Here's how the part is built. I have some questions about the finished solid (model axes, mm). A direction names the side the tool comes from. Give positions to 0.01 mm unless a question says otherwise; leave off trailing zeros. Write each loop counter-clockwise with the first axis right and the second up, starting at its lowest first coordinate (ties: lowest second). Pieces come first, ordered by that corner, then holes. Notation, with made-up numbers: (36.25, 73) -> (53.25, 73) arc R34 cw to (53.25, 110) -> close; hole circle Ø1 at (8, -25.75). An arc over 180 degrees is marked (long way). Return JSON: item names as keys, results as strings.
from build123d import *

# Parameters (mm, degrees)
CROQUIS1_W              = 5.7
CROQUIS1_H              = 2.6
SALIENTE_EXTRUIR1_DEPTH = 6.2
CROQUIS2_W              = 5.4
CROQUIS2_H              = 0.8
SALIENTE_EXTRUIR2_DEPTH = 1.4
SALIENTE_EXTRUIR3_DEPTH = 1
MATRIZL1_COUNT          = 2
MATRIZL1_PITCH          = 4.2


with BuildPart() as part:
    # Croquis1 → Saliente-Extruir1 (new body)
    with BuildSketch(Plane(origin=(0, 0, 0), x_dir=(0, 0, -1), z_dir=(1, 0, 0))):
        with Locations((2.85, 1.3)):
            Rectangle(CROQUIS1_W, CROQUIS1_H)
    extrude(amount=SALIENTE_EXTRUIR1_DEPTH)

    # Croquis2 → Saliente-Extruir2 (add)
    with BuildSketch(Plane.XY):
        with Locations((3.1, 0.4)):
            Rectangle(CROQUIS2_W, CROQUIS2_H)
    extrude(amount=SALIENTE_EXTRUIR2_DEPTH)

    # Croquis3 → Saliente-Extruir3 (add)
    with BuildSketch(Plane.ZY.offset(-0.5)):
        Polygon((-5.7, 1.8), (-6.3, 1.8), (-7.167456635, 0.5), (-8.7, 0.5), (-8.7, 0), (-6.9, 0), (-6.032543365, 1.3), (-5.7, 1.3), align=None)
    saliente_extruir3 = extrude(amount=-SALIENTE_EXTRUIR3_DEPTH)

    # MatrizL1: Saliente-Extruir3 ×2
    with Locations(*[(i * MATRIZL1_PITCH, 0, 0) for i in range(1, MATRIZL1_COUNT)]):
        add(saliente_extruir3)


solid = part.part
1. Suppose I cut it at B-B, the plane y = 0.2. List the corners of the cut face in (x, z) for me, and give its area (3 significant figures).
Taken from the geometry:
{"outline": "(0, -5.7) -> (6.2, -5.7) -> (6.2, 0) -> (5.8, 0) -> (5.8, 1.4) -> (0.4, 1.4) -> (0.4, 0) -> (0, 0) -> close; (0.5, -8.7) -> (1.5, -8.7) -> (1.5, -6.77) -> (0.5, -6.77) -> close; (4.7, -8.7) -> (5.7, -8.7) -> (5.7, -6.77) -> (4.7, -6.77) -> close", "area": "46.8 mm²"}
2. For pin 1 Ø0.8 at (x, y) = (4.5, 2) entering from +Z; pin 2 Ø1.4 at (y, z) = (1, -8) entering from +X; pin 3 Ø0.6 at (y, z) = (0.5, 1) entering from +X; pin 4 Ø0.5 at (y, z) = (1.5, -7) entering from +X, each with a flat end and sliding along its axis, tell me the tip position at first contact or that it passes through.
Taken from the geometry:
{"pin 1": "stops at z = 0", "pin 2": "stops at x = 5.7", "pin 3": "stops at x = 5.8", "pin 4": "passes through"}
3. Suppose I cut it at A-A, the plane z = -7.75. List the corners of the cut face in (x, y) for me, and give its area (3 significant figures).
Taken from the geometry:
{"outline": "(0.5, 0) -> (1.5, 0) -> (1.5, 0.5) -> (0.5, 0.5) -> close; (4.7, 0) -> (5.7, 0) -> (5.7, 0.5) -> (4.7, 0.5) -> close", "area": "1.00 mm²"}
4. If I drill on line 1 (X direction, y = 1.15, z = -6.5); line 2 (Z direction, x = 5.25, y = 2); line 3 (Z direction, x = 3, y = 0.5), over which ranges is the centre line in solid material (lowest first)? Write a range as [from, to].
Taken from the geometry:
{"line 1": "x = [0.5, 1.5], [4.7, 5.7]", "line 2": "z = [-5.7, 0]", "line 3": "z = [-5.7, 1.4]"}
5. If we mould it in two halves opening along X, with no side actions, what happens to faces 1 (the face through (1.5, 0.5, -6.98)), 2 (the face through (1, 1.2, -6.7)), 3 (the face through (0, 1, -3))? For each: released by +X, released by -X, zero draft, split by the parting line, or undercut.
Taken from the geometry:
{"face 1": "undercut", "face 2": "zero draft", "face 3": "released by -X"}
6. Suppose I cut it at C-C, the plane x = 3.5. List the corners of the cut face in (y, z) for me, and give its area (3 significant figures).
Taken from the geometry:
{"outline": "(0, -5.7) -> (2.6, -5.7) -> (2.6, 0) -> (0.8, 0) -> (0.8, 1.4) -> (0, 1.4) -> close", "area": "15.9 mm²"}
7. Suppose I cut it at D-D, the plane y = 2. List the corners of the cut face in (x, z) for me, and give its area (3 significant figures).
Taken from the geometry:
{"outline": "(0, -5.7) -> (6.2, -5.7) -> (6.2, 0) -> (0, 0) -> close", "area": "35.3 mm²"}
8. Which directions (+Z, -Z, +X, -X, +Y, -Y) give clear straight access to the entire face, cutting with the end or side of a thin tool? Please do faces 4 (the face through (1, 0.6, -6.5)), 5 (the face through (5.7, 0.5, -6.98)), 6 (the face through (4.7, 0.5, -6.98)), 7 (the face through (3, 0.8, 1)), 8 (the face through (1, 0.5, -8)).
Taken from the geometry:
{"face 4": "+X, -X, -Y", "face 5": "-Z, +X, +Y, -Y", "face 6": "-Z, +Y, -Y", "face 7": "+Z, +X, -X, +Y", "face 8": "-Z, +X, -X, +Y"}
